Source: CAD feature listing. Evaluate the final solid. Frame: model axes, mm. Coordinates: 2 decimals unless noted, no trailing zeros. Loops run counter-clockwise (first coordinate to the right, second up) from the corner with the lowest first, then second, coordinate; pieces in that order, holes last. Notation, with made-up numbers: M -40,9.5 L -16,9.5 A18 ccw -16,27.5 Z; hole C -26.5,44 d1. An arc over 180 degrees is marked long. One line per question, with ' | ' between items. Start each with the question number.
1. Pin query (flat end, axial travel): P1, Ø1.5, axis at x = 2.5, y = 3.5, coming from the -Z side. Return the tip coordinate at first contact, or that it passes through.
2. Section query A-A, the plane y = 7.25. Output: boundary loops of the cut face in (x, z), and give its area (3 significant figures).
3. Ray query, probe 1 along X at (y, z) = (7.5, -4.75); probe 2 along X at (y, z) = (6, 2.5); probe 3 along Z at (x, y) = (-24, 2.75). Return the intervals inside material, ascending.
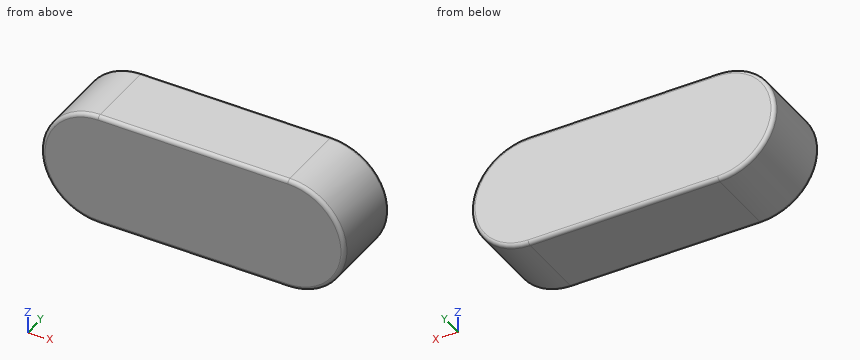
```python
from build123d import *

# Parameters (mm, degrees)
EXTRUDE1_DEPTH = 8
FILLET1_R      = 0.4


with BuildPart() as part:
    # Sketch1 → Extrude1 (new body)
    with BuildSketch(Plane(origin=(0, 0, 0), x_dir=(1, 0, 0), z_dir=(0, 1, 0))):
        with BuildLine():
            Line((-20, 6), (0, 6))
            ThreePointArc((0, 6), (6, 0), (0, -6))
            Line((0, -6), (-20, -6))
            ThreePointArc((-20, -6), (-26, 0), (-20, 6))
        make_face()
    extrude(amount=EXTRUDE1_DEPTH)

    # Fillet1
    fillet1_edges = [part.edges().sort_by_distance(p)[0] for p in [
        (6, 8, 0),
        (-10, 8, -6),
        (-26, 8, 0),
        (-10, 0, -6),
        (6, 0, 0),
        (-10, 0, 6),
        (-26, 0, 0),
        (-10, 8, 6),
    ]]
    fillet(fillet1_edges, radius=FILLET1_R)


solid = part.part
```
Taken from the geometry:
1) P1: z = -5.74
2) outline: M -20,-6 L 0,-6 A6 ccw 0,6 L -20,6 A6 ccw Z | area: 353 mm^2
3) probe 1: -23.67 to 3.67 | probe 2: -25.45 to 5.45 | probe 3: -4.47 to 4.47
